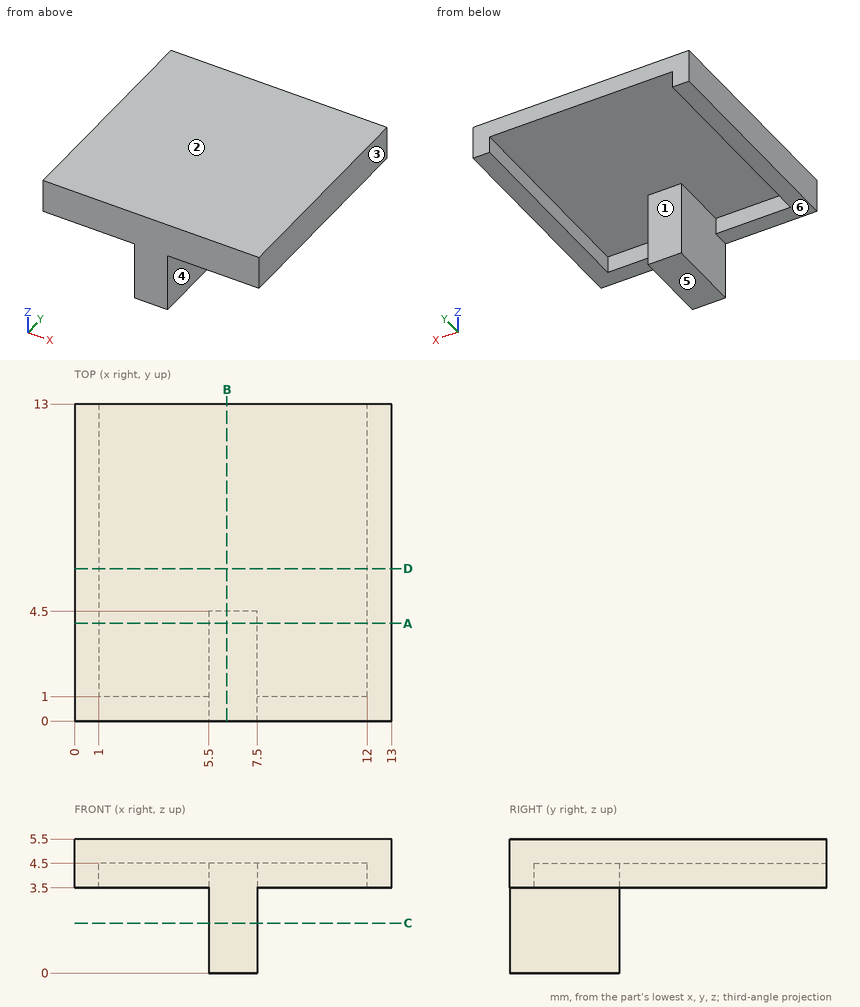
Verification items for this drawing (mm, ordinates from the low corner). A direction names the side the tool comes from. Round coordinates to 2 decimals unless told otherwise and drop trailing zeros. Order: outer loops, then holes, each group sorted by start corner. A loop starts at its lowest first (then second) coordinate and runs counter-clockwise, first axis right, second up. Notation, with made-up numbers: (48.25, 72.25) -> (100.25, 72.25) arc R21 cw to (100.25, 92.25) -> close; hole circle Ø11 at (54, -34.5). An arc over 180 degrees is marked (long way). Use one line per item in the form item = value.
1. Cross-section at C-C, the plane z = 2.05. Enter the section's corners in (x, y), plus the area to 3 significant figures.
Working result:
outline = (5.5, 0) -> (7.5, 0) -> (7.5, 4.5) -> (5.5, 4.5) -> close
area = 9.00 mm^2
2. Cross-section at B-B, the plane x = 6.25. Enter the section's corners in (y, z).
Working result:
outline = (0, 0) -> (4.5, 0) -> (4.5, 4.5) -> (13, 4.5) -> (13, 5.5) -> (0, 5.5) -> close
3. Set-up check for the marked faces 4, 5 and 6: record each of +Z, -Z, +X, -X, +Y, -Y from which the full face is reachable in a straight line by a thin tool's end or side.
Working result:
face_4 = -Z, +Y
face_5 = -Z, +X, -X, +Y, -Y
face_6 = -Z, -X, +Y, -Y
4. Go/stop test with flat-tipped pins: pin 1 (3 mm diameter, centred on y = 3, z = 1.5, fed in from -X); pin 2 (1 mm diameter, centred on x = 6.5, z = 1.5, fed in from +Y); pin 3 (0.8 mm diameter, centred on x = 9, z = 4, fed in from +Y). Record where each tip stops, or that it passes through.
Working result:
pin_1 = 5.5
pin_2 = 4.5
pin_3 = 1
5. Mould release check, pull along X, two halves, no side actions. Record for the marked faces 1, 2 and 3: pulls with the +X half, pulls with the -X half, needs draft (parallel to the pull), parting line crosses it, or undercut.
Working result:
face_1 = undercut
face_2 = needs draft
face_3 = pulls with the +X half
6. Cross-section at A-A, the plane y = 4. Enter the section's corners in (x, z), plus the area to 3 significant figures.
Working result:
outline = (0, 3.5) -> (1, 3.5) -> (1, 4.5) -> (5.5, 4.5) -> (5.5, 0) -> (7.5, 0) -> (7.5, 4.5) -> (12, 4.5) -> (12, 3.5) -> (13, 3.5) -> (13, 5.5) -> (0, 5.5) -> close
area = 24.0 mm^2
7. Cross-section at D-D, the plane y = 6.25. Enter the section's corners in (x, z), plus the area to 3 significant figures.
Working result:
outline = (0, 3.5) -> (1, 3.5) -> (1, 4.5) -> (12, 4.5) -> (12, 3.5) -> (13, 3.5) -> (13, 5.5) -> (0, 5.5) -> close
area = 15.0 mm^2
8. Scan lines: line 1 along X through (y, z) = (2, 3.65); line 2 along X through (y, z) = (6.75, 3.6); line 3 along X through (y, z) = (3.5, 2.1). Record each from-to range of solid material in increasing order. Write a range as from..to.
Working result:
line_1 = 0..1, 5.5..7.5, 12..13
line_2 = 0..1, 12..13
line_3 = 5.5..7.5
